from build123d import *

# Parameters (mm, degrees)
F2_W     = 15.68
F2_H     = 15.68
F2_W_2   = 13.24
F2_H_2   = 13.24
F3_DEPTH = 5
F2_R     = 3.25
F2_R_2   = 2.25
F5_W     = 15.68
F5_H     = 15.68
F6_DEPTH = 2.5
F7_R     = 2.435
F8_DEPTH = 1.9


with BuildPart() as f3:
    # F2 (on Top) → F3 (new body)
    with BuildSketch(Plane.XY):
        Rectangle(F2_W, F2_H)
        Rectangle(F2_W_2, F2_H_2, mode=Mode.SUBTRACT)
    extrude(amount=F3_DEPTH)



with BuildPart() as f3b:
    # F2 (on Top) → F3, piece 2 (new body)
    with BuildSketch(Plane.XY):
        Circle(F2_R)
        Circle(F2_R_2, mode=Mode.SUBTRACT)
    extrude(amount=F3_DEPTH)


with BuildPart() as f3_1:
    add(f3.part)

    add(f3b.part)  # F6 merges F3b
    # F5 (on offset) → F6 (join)
    with BuildSketch(Plane.XY.offset(5)):
        Rectangle(F5_W, F5_H)
    extrude(amount=F6_DEPTH)

    # F7 (on face) → F8 (join)
    with BuildSketch(Plane.XY.offset(7.5)):
        with Locations((-3.9575, 3.9575)):
            Circle(F7_R)
        with Locations((-3.9575, -3.9575)):
            Circle(F7_R)
        with Locations((3.9575, -3.9575)):
            Circle(F7_R)
        with Locations((3.9575, 3.9575)):
            Circle(F7_R)
    extrude(amount=F8_DEPTH)


solid = f3_1.part
Geometry: final body of the model. Coordinates: model frame, mm. A direction names the side the tool comes from. Coordinates: 2 decimals unless noted, no trailing zeros. Loops run counter-clockwise (first coordinate to the right, second up) from the corner with the lowest first, then second, coordinate; pieces in that order, holes last. Notation, with made-up numbers: (-33.5, 8) - (-18.5, 8) arc R24 ccw to (-18.5, 36) - close; hole circle Ø11 at (19, 57). An arc over 180 degrees is marked (long way). Put each result on its own line as item: value. Start each with the question number.
Q1. Pin query (flat end, axial travel): pin 1 Ø2 at (x, y) = (-1, -0.5) entering from -Z. Return the tip coordinate at first contact, or that it passes through.
Q2. Cut plane A-A, the plane z = 0.5. Return loops of the section in (x, y).
Q3. Cut plane D-D, the plane z = 8.5. Return loops of the section in (x, y) (1 decimal).
Q4. Pull-direction query (Y, two-part tool) for faces 4 (the flat face through (0, 7.84, 4)), 5 (the flat face through (4, 4, 9.4)), 6 (the flat face through (0, -6.62, 2)); classes: released by +Y, released by -Y, zero draft, split by the parting line, or undercut.
Q5. Cut plane B-B, the plane y = 0. Return loops of the section in (x, z), and give its area (3 significant figures).
Q6. Set-up query: faces 1 (the flat face through (6.62, 0, 2)), 2 (the cylindrical face through (6.28, -3.23, 8.44)), 3 (the flat face through (0, -7.84, 4)). Return all of +Z, -Z, +X, -X, +Y, -Y with unobstructed straight access to the full face (end or side cutting, diameter ignored); none if empty.
Q7. Line query: line 1 (Y direction, x = 0, z = 2.75); line 2 (X direction, y = -1.5, z = 1); line 3 (Y direction, x = -3.75, z = 4.75). Output: solid intervals per line, ascending.
Filled sheet:
1. pin 1: z = 5
2. outline: (-7.84, -7.84) - (7.84, -7.84) - (7.84, 7.84) - (-7.84, 7.84) - close; circle Ø6.5 at (0, 0); hole (-6.62, -6.62) - (6.62, -6.62) - (6.62, 6.62) - (-6.62, 6.62) - close; hole circle Ø4.5 at (0, 0)
3. outline: circle Ø4.9 at (-4, -4); circle Ø4.9 at (-4, 4); circle Ø4.9 at (4, -4); circle Ø4.9 at (4, 4)
4. face 4: released by +Y
4. face 5: zero draft
4. face 6: undercut
5. outline: (-7.84, 0) - (-6.62, 0) - (-6.62, 5) - (-3.25, 5) - (-3.25, 0) - (-2.25, 0) - (-2.25, 5) - (2.25, 5) - (2.25, 0) - (3.25, 0) - (3.25, 5) - (6.62, 5) - (6.62, 0) - (7.84, 0) - (7.84, 7.5) - (-7.84, 7.5) - close
5. area: 61.4 mm²
6. face 1: -Z
6. face 2: +Z
6. face 3: +Z, -Z, +X, -X, -Y
7. line 1: -7.84 to -6.62, -3.25 to -2.25, 2.25 to 3.25, 6.62 to 7.84
7. line 2: -7.84 to -6.62, -2.88 to -1.68, 1.68 to 2.88, 6.62 to 7.84
7. line 3: -7.84 to -6.62, 6.62 to 7.84
